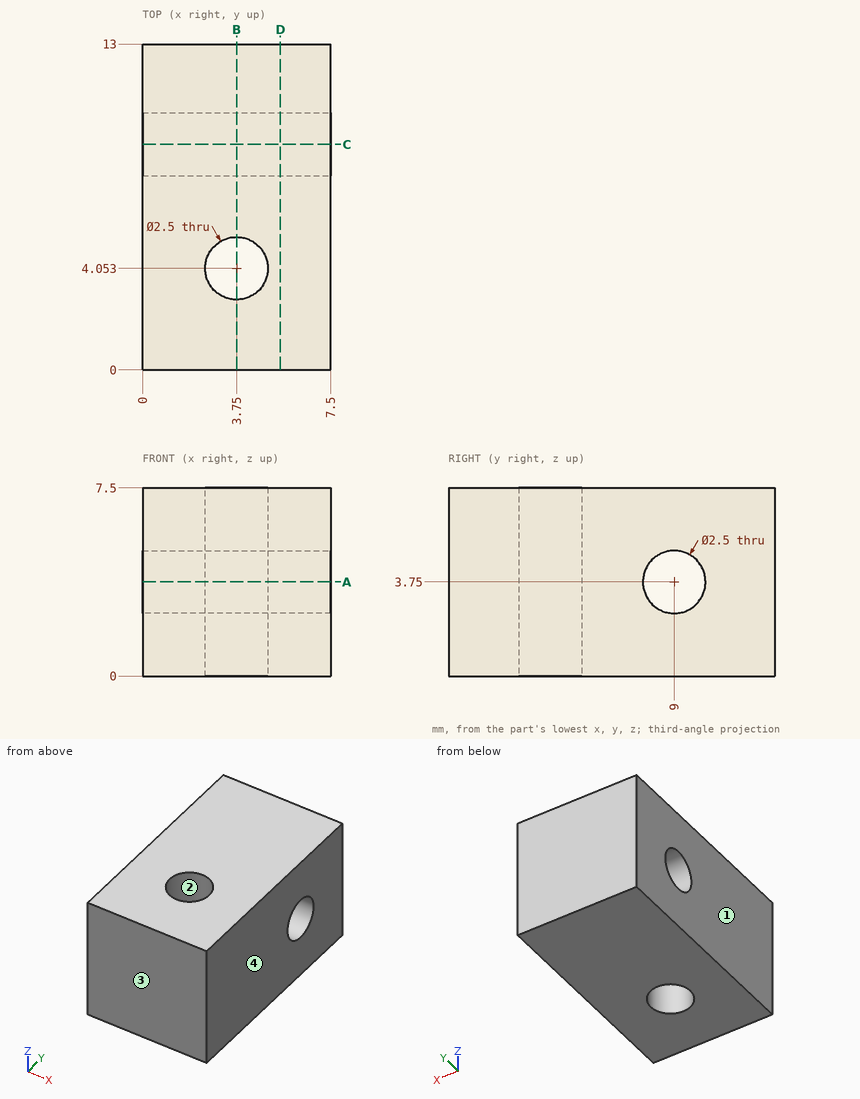
For this review, use the dimensioned drawing (mm, ordinates from the lowest corner) and the shaded views. Round coordinates to 2 decimals unless told otherwise and drop trailing zeros. Write each loop counter-clockwise with the first axis right and the second up, starting at its lowest first coordinate (ties: lowest second). Pieces come first, ordered by that corner, then holes. Notation, with made-up numbers: (2, 54) - (12, 54) arc R30 ccw to (12, 87) - close; hole circle Ø4 at (-30, 23). An arc over 180 degrees is marked (long way). Answer as a JSON object with one key per item and string values.
1. We need section D-D on x = 5.5. Give the boundary of the cut face in (y, z), then the cut area to 3 significant figures.
Response values:
{"outline": "(0, 0) - (13, 0) - (13, 7.5) - (0, 7.5) - close; hole circle Ø2.5 at (9, 3.75)", "area": "92.6 mm2"}
2. Draft analysis for pull direction X (two halves, no side actions). For the marked faces 1, 2, 3 and 4, state which applies: +X half, -X half, draft (parallel to the pull), parting line (faces both ways), or undercut.
Response values:
{"face 1": "-X half", "face 2": "undercut", "face 3": "draft", "face 4": "+X half"}
3. We need section B-B on x = 3.75. Give the boundary of the cut face in (y, z), then the cut area to 3 significant figures.
Response values:
{"outline": "(0, 0) - (2.8, 0) - (2.8, 7.5) - (0, 7.5) - close; (5.3, 0) - (13, 0) - (13, 7.5) - (5.3, 7.5) - close; hole circle Ø2.5 at (9, 3.75)", "area": "73.8 mm2"}
4. For pin 1 Ø2 at (y, z) = (9, 3.75) entering from +X, flat-tipped, find the tip position at first contact; note if it passes through.
Response values:
{"pin 1": "passes through"}
5. We need section A-A on z = 3.75. Give the boundary of the cut face in (x, y).
Response values:
{"outline": "(0, 0) - (7.5, 0) - (7.5, 7.75) - (0, 7.75) - close; (0, 10.25) - (7.5, 10.25) - (7.5, 13) - (0, 13) - close; hole circle Ø2.5 at (3.75, 4.05)"}
6. We need section C-C on y = 9. Give the boundary of the cut face in (x, z).
Response values:
{"outline": "(0, 0) - (7.5, 0) - (7.5, 2.5) - (0, 2.5) - close; (0, 5) - (7.5, 5) - (7.5, 7.5) - (0, 7.5) - close"}
7. To check wall thickness, follow line 1 along Y through (x, z) = (5.5, 3.75); line 2 along Y through (x, z) = (3.5, 3.75); line 3 along Y through (x, z) = (3.25, 3.75). State the ranges of each line that lie inside material, in increasing order.
Response values:
{"line 1": "y = 0 to 7.75, 10.25 to 13", "line 2": "y = 0 to 2.83, 5.28 to 7.75, 10.25 to 13", "line 3": "y = 0 to 2.91, 5.2 to 7.75, 10.25 to 13"}
